Verification items for the finished model (mm, model axes). Face numbers are marked on the shaded views. A direction names the side the tool comes from. Round coordinates to 2 decimals unless told otherwise and drop trailing zeros. Order: outer loops, then holes, each group sorted by start corner. A loop starts at its lowest first (then second) coordinate and runs counter-clockwise, first axis right, second up. Notation, with made-up numbers: M -15.75,2.25 L 3.25,2.25 A19 cw 3.25,10.25 Z; hole C 14,60.5 d2. An arc over 180 degrees is marked long. Use CSV: the item, a comma, the result in double quotes. Start each with the question number.
Q1. Set-up check for the marked faces 4, 5 and 6: record each of +Z, -Z, +X, -X, +Y, -Y from which the full face is reachable in a straight line by a thin tool's end or side.
Q2. Sectioned sample at A-A (z = 8). Enter the section's corners in (x, y), and give its area (3 significant figures).
Q3. Sectioned sample at D-D (z = 39). Enter the section's corners in (x, y).
Q4. Sectioned sample at B-B (x = -9.5). Enter the section's corners in (y, z).
Q5. Gauge pin test, flat ends, axial feed: pin 1 Ø12.5 at (x, y) = (31.5, 9.5) entering from +Z; pin 2 Ø10 at (x, z) = (9.5, 11.5) entering from -Y; pin 3 Ø4 at (y, z) = (8.5, 44.5) entering from +X. Record the tip position at first contact, or that the pin passes through.
Q6. Sectioned sample at C-C (y = -5). Enter the section's corners in (x, z), and give its area (3 significant figures).
Q7. Scan lines: line 1 (Y direction, x = 6, z = 20); line 2 (X direction, y = 21.5, z = 44.5); line 3 (Z direction, x = -3, y = -5.5). Record each from-to range of solid material in increasing order.
Q8. Mould release check, pull along Y, two halves, no side actions. Record for the marked faces 1, 2 and 3: +Y half, -Y half, draft (parallel to the pull), parting line (faces both ways), or undercut.
```python
from build123d import *

# Parameters (mm, degrees)
F0_W     = 76.2
F0_H     = 25.4
F1_DEPTH = 38.1
F2_W     = 38.1
F2_H     = 25.4
F3_DEPTH = 25.4
F4_W     = 50.8
F4_H     = 25.4
F5_DEPTH = 12.7


with BuildPart() as f1:
    # F0 (on Top) → F1 (new body)
    with BuildSketch(Plane.XY):
        with Locations((1.447711, 12.8482)):
            Rectangle(F0_W, F0_H)
    extrude(amount=F1_DEPTH)

    # F2 (on face) → F3 (join)
    with BuildSketch(Plane.XZ.offset(-0.1482)):
        with Locations((-17.602289, 12.7)):
            Rectangle(F2_W, F2_H)
    extrude(amount=F3_DEPTH)

    # F4 (on face) → F5 (join)
    with BuildSketch(Plane.XY.offset(38.1)):
        with Locations((-11.252289, 12.8482)):
            Rectangle(F4_W, F4_H)
    extrude(amount=F5_DEPTH)


solid = f1.part
```
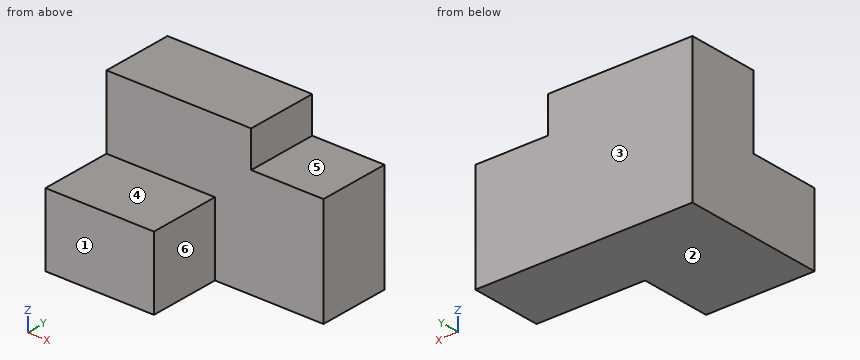
Verdict:
1,face 4,"+Z, +X, -X, -Y"
1,face 5,"+Z, +X, +Y, -Y"
1,face 6,"+Z, -Z, +X, -Y"
2,outline,"M -36.65,-25.25 L 1.45,-25.25 L 1.45,0.15 L 39.55,0.15 L 39.55,25.55 L -36.65,25.55 Z"
2,area,"2,900 mm²"
3,outline,"M -36.65,0.15 L 14.15,0.15 L 14.15,25.55 L -36.65,25.55 Z"
4,outline,"M -25.25,0 L 25.55,0 L 25.55,50.8 L 0.15,50.8 L 0.15,25.4 L -25.25,25.4 Z"
5,pin 1,"stops at z = 38.1"
5,pin 2,"stops at y = 0.15"
5,pin 3,"stops at x = 14.15"
6,outline,"M -36.65,0 L 1.45,0 L 1.45,25.4 L -36.65,25.4 Z"
6,area,"968 mm²"
7,line 1,"y = 0.15 to 25.55"
7,line 2,"x = -36.65 to 14.15"
7,line 3,"z = 0 to 25.4"
8,face 1,"-Y half"
8,face 2,"draft"
8,face 3,"+Y half"
